```python
from build123d import *

# Parameters (mm, degrees)
ESQUISSE1_R        = 2.1
BOSS_EXTRU_1_DEPTH = 5


with BuildPart() as part:
    # Esquisse1 → Boss.-Extru.1 (new body)
    with BuildSketch(Plane.XY):
        with BuildLine():
            Line((-78.135883383, 18.842375861), (-83.135883383, 18.842375861))
            Line((-83.135883383, 18.842375861), (-83.135883383, 23.843375961))
            ThreePointArc((-83.135883383, 23.843375961), (-84.935883383, 28.128233018), (-83.135883383, 32.413090075))
            ThreePointArc((-83.135883383, 32.413090075), (-76.612093375, 33.659959692), (-72.935883383, 28.128233018))
            Line((-72.935883383, 28.128233018), (0, 28.128233018))
            Line((0, 28.128233018), (0, 13.842375861))
            Line((0, 13.842375861), (0, -31.157624139))
            Line((0, -31.157624139), (-30, -31.157624139))
            ThreePointArc((-30, -31.157624139), (-51.303897557, -7.472735951), (-77.105155917, -26.157624139))
            Line((-77.105155917, -26.157624139), (-83.135883383, -26.157624139))
            Line((-83.135883383, -26.157624139), (-83.135883383, -16.157624139))
            Line((-83.135883383, -16.157624139), (-78.135883383, -16.157624139))
            Line((-78.135883383, -16.157624139), (-78.135883383, -11.157624139))
            Line((-78.135883383, -11.157624139), (-83.135883383, -11.157624139))
            Line((-83.135883383, -11.157624139), (-83.135883383, -6.157624139))
            Line((-83.135883383, -6.157624139), (-78.135883383, -6.157624139))
            Line((-78.135883383, -6.157624139), (-78.135883383, -1.157624139))
            Line((-78.135883383, -1.157624139), (-83.135883383, -1.157624139))
            Line((-83.135883383, -1.157624139), (-83.135883383, 3.842375861))
            Line((-83.135883383, 3.842375861), (-78.135883383, 3.842375861))
            Line((-78.135883383, 3.842375861), (-78.135883383, 8.842375861))
            Line((-78.135883383, 8.842375861), (-83.135883383, 8.842375861))
            Line((-83.135883383, 8.842375861), (-83.135883383, 13.842375861))
            Line((-83.135883383, 13.842375861), (-78.135883383, 13.842375861))
            Line((-78.135883383, 13.842375861), (-78.135883383, 18.842375861))
        make_face()
        with Locations((-78.935883383, 28.128233018)):
            Circle(ESQUISSE1_R, mode=Mode.SUBTRACT)
    extrude(amount=BOSS_EXTRU_1_DEPTH)


solid = part.part
```
Source: CAD feature listing. Evaluate the final solid. Frame: model axes, mm. A direction names the side the tool comes from. Coordinates: 2 decimals unless noted, no trailing zeros. Loops run counter-clockwise (first coordinate to the right, second up) from the corner with the lowest first, then second, coordinate; pieces in that order, holes last. Notation, with made-up numbers: M -36.75,-7 L -9.75,-7 A32 ccw -9.75,24 Z; hole C -12,40 d11. An arc over 180 degrees is marked long. Put each result on its own line as item: value. Start each with the question number.
1) Cut plane C-C on x = -24. Return the cut outline in (y, z).
2) Cut plane B-B on z = 3.1. Return the cut outline in (x, y), then the cut area to 3 significant figures.
3) Pull-direction query (Y, two-part tool) for faces 4 (the face through (-50.82, -7.53, 2.46)), 5 (the face through (-81, -6.158, 2)), 6 (the face through (-37, 28.128, 2)), 7 (the face through (-83.136, -9, 2)); classes: pulls with the +Y half, pulls with the -Y half, needs draft (parallel to the pull), parting line crosses it, or undercut.
4) Contact query for flat-ended pins moving along their axis: pin 1 Ø1.5 at (y, z) = (15.5, 3.5) entering from -X; pin 2 Ø2.5 at (x, z) = (-79.5, 2) entering from -Y; pin 3 Ø2.5 at (x, z) = (-80.5, 3) entering from +Y. Output: stop coordinate, or through.
5) Cut plane D-D on y = 7.5. Return the cut outline in (x, z).
6) Cut plane A-A on y = -15. Return the cut outline in (x, z).
7) Reachability of faces 1 (the face through (-81, -1.158, 2)), 2 (the face through (-42, 2, 5)), 3 (the face through (-83.136, 11, 2)) from +Z, -Z, +X, -X, +Y, -Y: full face, straight path, thin tool, end or side. Return the list, or none.
8) Ray query, L1, parallel to Y at x = -79, z = 4.5; L2, parallel to X at y = 4, z = 4.85; L3, parallel to X at y = -18.5, z = 3.05. Return the intervals inside material, ascending. Write a range as from..to.
The answers:
1. outline: M -31.16,0 L 28.13,0 L 28.13,5 L -31.16,5 Z
2. outline: M -83.14,-26.16 L -77.11,-26.16 A23.82 cw -30,-31.16 L 0,-31.16 L 0,28.13 L -72.94,28.13 A6 ccw long -83.14,23.84 L -83.14,18.84 L -78.14,18.84 L -78.14,13.84 L -83.14,13.84 L -83.14,8.84 L -78.14,8.84 L -78.14,3.84 L -83.14,3.84 L -83.14,-1.16 L -78.14,-1.16 L -78.14,-6.16 L -83.14,-6.16 L -83.14,-11.16 L -78.14,-11.16 L -78.14,-16.16 L -83.14,-16.16 Z; hole C -78.94,28.13 d4.2
2. area: 3,960 mm²
3. face 4: pulls with the -Y half
3. face 5: undercut
3. face 6: pulls with the +Y half
3. face 7: needs draft
4. pin 1: stops at x = -78.14
4. pin 2: stops at y = -26.16
4. pin 3: stops at y = 34.12
5. outline: M -78.14,0 L 0,0 L 0,5 L -78.14,5 Z
6. outline: M -78.14,0 L -71.32,0 L -71.32,5 L -78.14,5 Z; M -36.32,0 L 0,0 L 0,5 L -36.32,5 Z
7. face 1: +Z, -Z, -X
7. face 2: +Z, +X, -X, +Y, -Y
7. face 3: +Z, -Z, -X, -Y
8. L1: y = -26.16..-16.16, -11.16..-6.16, -1.16..3.84, 8.84..13.84, 18.84..26.03, 30.23..34.13
8. L2: x = -78.14..0
8. L3: x = -83.14..-73.99, -33.64..0
